```python
from build123d import *

# Parameters (mm, degrees)
SKICA1_R                 = 6
P_IDAT_VYSUNUT_M1_DEPTH  = 7
SKICA5_R                 = 6
SKICA5_R_2               = 4
P_IDAT_VYSUNUT_M3_DEPTH  = 5
SKICA6_R                 = 6
P_IDAT_VYSUNUT_M4_DEPTH  = 0.6
SKICA7_R                 = 1.266795128
P_IDAT_VYSUNUT_M5_DEPTH  = 1
SKICA8_R                 = 1.792460028
ODEBRAT_VYSUNUT_M2_DEPTH = 21
ODEBRAT_VYSUNUT_M4_DEPTH = 7
P_IDAT_VYSUNUT_M6_DEPTH  = 0.5
P_IDAT_VYSUNUT_M7_DEPTH  = 5


with BuildPart() as part:
    # Skica1 → Přidat vysunutím1 (new body)
    with BuildSketch(Plane.XY):
        Circle(SKICA1_R)
        with BuildLine():
            Line((-2.524876235, -1.575), (2.524876235, -1.575))
            ThreePointArc((2.524876235, -1.575), (2.627027018, -1.546945391), (2.700519799, -1.470652174))
            ThreePointArc((2.700519799, -1.470652174), (0, 3.075), (-2.700519799, -1.470652174))
            ThreePointArc((-2.700519799, -1.470652174), (-2.627027018, -1.546945391), (-2.524876235, -1.575))
        make_face(mode=Mode.SUBTRACT)
    extrude(amount=P_IDAT_VYSUNUT_M1_DEPTH)

    # Skica5 → Přidat vysunutím3 (add)
    with BuildSketch(Plane.XY.offset(7)):
        Circle(SKICA5_R)
        Circle(SKICA5_R_2, mode=Mode.SUBTRACT)
    extrude(amount=P_IDAT_VYSUNUT_M3_DEPTH)

    # Skica6 → Přidat vysunutím4 (add)
    with BuildSketch(Plane(origin=(0, 0, 0), x_dir=(-1, 0, 0), z_dir=(0, 0, -1))):
        Circle(SKICA6_R)
    extrude(amount=P_IDAT_VYSUNUT_M4_DEPTH)

    # Skica7 → Přidat vysunutím5 (add)
    with BuildSketch(Plane.XY.offset(5)):
        with Locations((0, -2.741795128)):
            Circle(SKICA7_R)
    extrude(amount=-P_IDAT_VYSUNUT_M5_DEPTH)

    # Skica8 → Odebrat vysunutím2 (cut)
    with BuildSketch(Plane.XY.offset(12)):
        with Locations((0, 7.222215072)):
            Circle(SKICA8_R)
        with Locations((4.642350363, 5.532537723)):
            Circle(SKICA8_R)
        with Locations((7.112493397, 1.254124486)):
            Circle(SKICA8_R)
        with Locations((6.254621724, -3.611107536)):
            Circle(SKICA8_R)
        with Locations((2.470143034, -6.786662209)):
            Circle(SKICA8_R)
        with Locations((-2.470143034, -6.786662209)):
            Circle(SKICA8_R)
        with Locations((-6.254621724, -3.611107536)):
            Circle(SKICA8_R)
        with Locations((-7.112493397, 1.254124486)):
            Circle(SKICA8_R)
        with Locations((-4.642350363, 5.532537723)):
            Circle(SKICA8_R)
    extrude(amount=-ODEBRAT_VYSUNUT_M2_DEPTH, mode=Mode.SUBTRACT)

    # Skica11 → Odebrat vysunutím4 (cut)
    with BuildSketch(Plane.XY.offset(7)):
        with BuildLine():
            Line((-2.524876235, -1.645), (2.524876235, -1.645))
            ThreePointArc((2.524876235, -1.645), (2.662779793, -1.607126277), (2.761995046, -1.504130435))
            ThreePointArc((2.761995046, -1.504130435), (0, 3.145), (-2.761995046, -1.504130435))
            ThreePointArc((-2.761995046, -1.504130435), (-2.662779793, -1.607126277), (-2.524876235, -1.645))
        make_face()
    extrude(amount=-ODEBRAT_VYSUNUT_M4_DEPTH, mode=Mode.SUBTRACT)

    # Skica12 → Přidat vysunutím6 (add, symmetric)
    with BuildSketch(Plane(origin=(0, 0, 0), x_dir=(0, 0, -1), z_dir=(1, 0, 0))):
        Polygon((-2, -1.645), (0, -1.495), (0, -1.645), align=None)
    extrude(amount=P_IDAT_VYSUNUT_M6_DEPTH, both=True)

    # Skica13 → Přidat vysunutím7 (add)
    with BuildSketch(Plane(origin=(0, 0, -0.6), x_dir=(-1, 0, 0), z_dir=(0, 0, -1))):
        with BuildLine():
            ThreePointArc((2.869302785, 5.269449832), (3.490179266, 4.159433679), (4.691145849, 3.740741989))
            ThreePointArc((4.691145849, 3.740741989), (5.196152423, 3), (5.585150516, 2.192280483))
            ThreePointArc((5.585150516, 2.192280483), (5.347264864, 0.942867069), (5.998128811, -0.149835813))
            ThreePointArc((5.998128811, -0.149835813), (5.908846518, -1.041889066), (5.687644248, -1.910681268))
            ThreePointArc((5.687644248, -1.910681268), (4.702305805, -2.714877522), (4.498520641, -3.970303773))
            ThreePointArc((4.498520641, -3.970303773), (3.856725658, -4.596266659), (3.128826026, -5.119614019))
            ThreePointArc((3.128826026, -5.119614019), (1.857085598, -5.102300748), (0.894004667, -5.933022472))
            ThreePointArc((0.894004667, -5.933022472), (0, -6), (-0.894004667, -5.933022472))
            ThreePointArc((-0.894004667, -5.933022472), (-1.857085598, -5.102300748), (-3.128826026, -5.119614019))
            ThreePointArc((-3.128826026, -5.119614019), (-3.856725658, -4.596266659), (-4.498520641, -3.970303773))
            ThreePointArc((-4.498520641, -3.970303773), (-4.702305805, -2.714877522), (-5.687644248, -1.910681268))
            ThreePointArc((-5.687644248, -1.910681268), (-5.908846518, -1.041889066), (-5.998128811, -0.149835813))
            ThreePointArc((-5.998128811, -0.149835813), (-5.347264864, 0.942867069), (-5.585150516, 2.192280483))
            ThreePointArc((-5.585150516, 2.192280483), (-5.196152423, 3), (-4.691145849, 3.740741989))
            ThreePointArc((-4.691145849, 3.740741989), (-3.490179266, 4.159433679), (-2.869302785, 5.269449832))
            ThreePointArc((-2.869302785, 5.269449832), (-2.05212086, 5.638155725), (-1.189123608, 5.88098504))
            ThreePointArc((-1.189123608, 5.88098504), (0, 5.429755044), (1.189123608, 5.88098504))
            ThreePointArc((1.189123608, 5.88098504), (2.05212086, 5.638155725), (2.869302785, 5.269449832))
        make_face()
    extrude(amount=P_IDAT_VYSUNUT_M7_DEPTH)

    # Skica14 → Odebrat rotací1 (revolve, cut)
    with BuildSketch(Plane(origin=(0, 0, 0), x_dir=(1, 0, 0), z_dir=(0, 1, 0))):
        Polygon((-0.519399501, 11.540173112), (-8.873937642, -0.391343881), (-8.306128357, 8.726101498), align=None)
    revolve(axis=Axis((0, 0, 0), (0, 0, -1)), mode=Mode.SUBTRACT)


solid = part.part
```
Geometry check sheet. Reference: the model listing, model coordinates, mm. A direction names the side the tool comes from. Round coordinates to 2 decimals unless told otherwise and drop trailing zeros. Order: outer loops, then holes, each group sorted by start corner. A loop starts at its lowest first (then second) coordinate and runs counter-clockwise, first axis right, second up. Notation, with made-up numbers: (41.25, 85) - (46.25, 85) arc R24 cw to (46.25, 109) - close; hole circle Ø10 at (62, 66). An arc over 180 degrees is marked (long way). Use a Markdown table: item, result. Add a question column.
(1) Material ranges on line 1 along Z through (x, y) = (2, 2); line 2 along X through (y, z) = (-0.75, 10); line 3 along X through (y, z) = (0, 2.25) (3 decimals), recorded low to high. Write a range as [from, to].
(2) Sectioned sample at B-B, the plane x = 0. Enter the section's corners in (y, z) (3 decimals).
(3) Sectioned sample at C-C, the plane z = -3.5. Enter the section's corners in (x, y), and give its area (3 significant figures).
(4) Sectioned sample at A-A, the plane z = 10.25. Enter the section's corners in (x, y).
(5) Tool access check on faces 1 (the flat face through (0, 0, -5.6)), 2 (the cylindrical face through (0.091, 3.144, 3.549)). Record the directions out of +Z, -Z, +X, -X, +Y, -Y that give a thin tool (end or side, any length) a straight path to the whole face; none if there is none.
(6) Release check for a two-part mould opening along X. For faces 3 (the flat face through (1.2, 4, 12)), 4 (the flat face through (0, -1.645, 4)), 5 (the conical face through (-5, 1, -5)) record: pulls with the +X half, pulls with the -X half, needs draft (parallel to the pull), parting line crosses it, or undercut.
(7) Depth check by flat-ended pin: pin 1 (2 mm diameter, centred on x = 2, y = 2, fed in from +Z); pin 2 (3 mm diameter, centred on x = -4, z = 4.5, fed in from -Y); pin 3 (1 mm diameter, centred on y = -1.5, z = 6.5, fed in from -X). Enter the tip coordinate at first touch or a pass-through.
Answers below:
| question | item | result |
|---|---|---|
| 1 | line 1 | [-5.6, 0] |
| 1 | line 2 | [-5.95, -3.93], [3.93, 5.95] |
| 1 | line 3 | [-5.832, -3.145], [3.145, 5.832] |
| 2 | outline | (-6, -3.713) - (-4.679, -5.6) - (4.679, -5.6) - (5.43, -4.527) - (5.43, 12) - (4, 12) - (4, 7) - (3.145, 7) - (3.145, 0) - (-1.495, 0) - (-1.645, 2) - (-1.645, 7) - (-4, 7) - (-4, 12) - (-6, 12) - close |
| 3 | outline | (-6, -0.15) arc R6 ccw to (-5.69, -1.91) arc R1.79 cw to (-4.5, -3.97) arc R6 ccw to (-3.13, -5.12) arc R1.79 cw to (-0.89, -5.93) arc R6 ccw to (0.89, -5.93) arc R1.79 cw to (3.13, -5.12) arc R6 ccw to (4.5, -3.97) arc R1.79 cw to (5.69, -1.91) arc R6 ccw to (6, -0.15) arc R1.79 cw to (5.59, 2.19) arc R6 ccw to (4.69, 3.74) arc R1.79 cw to (2.87, 5.27) arc R6 ccw to (1.19, 5.88) arc R1.79 cw to (-1.19, 5.88) arc R6 ccw to (-2.87, 5.27) arc R1.79 cw to (-4.69, 3.74) arc R6 ccw to (-5.59, 2.19) arc R1.79 cw to start |
| 3 | area | 105 mm² |
| 4 | outline | (-6, -0.15) arc R6 ccw to (-5.69, -1.91) arc R1.79 cw to (-4.5, -3.97) arc R6 ccw to (-3.13, -5.12) arc R1.79 cw to (-0.89, -5.93) arc R6 ccw to (0.89, -5.93) arc R1.79 cw to (3.13, -5.12) arc R6 ccw to (4.5, -3.97) arc R1.79 cw to (5.69, -1.91) arc R6 ccw to (6, -0.15) arc R1.79 cw to (5.59, 2.19) arc R6 ccw to (4.69, 3.74) arc R1.79 cw to (2.87, 5.27) arc R6 ccw to (1.19, 5.88) arc R1.79 cw to (-1.19, 5.88) arc R6 ccw to (-2.87, 5.27) arc R1.79 cw to (-4.69, 3.74) arc R6 ccw to (-5.59, 2.19) arc R1.79 cw to start; hole circle Ø8 at (0, 0) |
| 5 | face 1 | -Z, +X, -X, +Y, -Y |
| 5 | face 2 | +Z |
| 6 | face 3 | needs draft |
| 6 | face 4 | undercut |
| 6 | face 5 | parting line crosses it |
| 7 | pin 1 | z = 7 |
| 7 | pin 2 | y = -5.12 |
| 7 | pin 3 | x = -5.92 |
